Read the model definition and answer for the solid it produces. Units are mm, in the model's axes. Face numbers are marked on the shaded views. A direction names the side the tool comes from. Coordinates: 2 decimals unless noted, no trailing zeros. Loops run counter-clockwise (first coordinate to the right, second up) from the corner with the lowest first, then second, coordinate; pieces in that order, holes last.
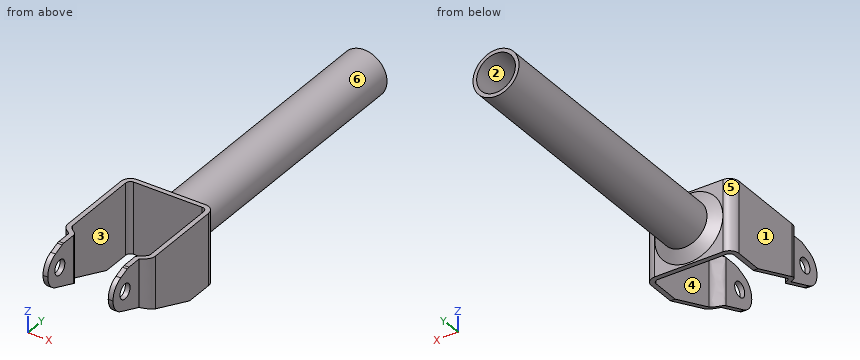
from build123d import *

# Parameters (mm, degrees)
EXTRUDE_THIN1_DEPTH = 38.1
CUT_EXTRUDE1_DEPTH  = 96.205221294
SKETCH5_R           = 3.96875
CUT_EXTRUDE2_DEPTH  = 96.205221294
SKETCH6_R           = 12.2936
SKETCH6_R_2         = 10.342534733
BOSS_EXTRUDE2_DEPTH = 152.4
SKETCH8_R           = 18.199007784
SKETCH7_R           = 10.342534733


# Read off the part's stored shape, not the designer's step: Extrude-Thin1
with BuildPart() as part:
    # Extrude-Thin1 outline → Extrude-Thin1 (new body)
    with BuildSketch(Plane.XY):
        with BuildLine():
            Line((-18.6817, 20.38347688), (-18.6817, 0))
            Line((-18.6817, 0), (-16.1417, 0))
            Line((-16.1417, 0), (-16.1417, 20.32))
            add(Edge.make_bspline(
                [(-20.8407, 26.67), (-20.8407, 23.763857752), (-15.646351535, 22.789211476), (-16.1417, 20.32)],
                knots=[0, 0, 0, 0, 1, 1, 1, 1], degree=3))
            Line((-20.8407, 26.67), (-20.8407, 68.58))
            ThreePointArc((-20.8407, 68.58), (-20.096751224, 70.376051224), (-18.3007, 71.12))
            Line((-18.3007, 71.12), (18.3007, 71.12))
            ThreePointArc((18.3007, 71.12), (20.096751224, 70.376051224), (20.8407, 68.58))
            Line((20.8407, 68.58), (20.8407, 26.67))
            add(Edge.make_bspline(
                [(16.1417, 20.32), (15.646351535, 22.789211476), (20.8407, 23.763857752), (20.8407, 26.67)],
                knots=[0, 0, 0, 0, 1, 1, 1, 1], degree=3))
            Line((16.1417, 20.32), (16.1417, 0))
            Line((16.1417, 0), (18.6817, 0))
            Line((18.6817, 0), (18.6817, 20.38347688))
            add(Edge.make_bspline(
                [(18.6817, 20.38347688), (18.765268898, 20.466690468), (18.888895007, 20.57668849), (19.198318415, 20.827254502), (19.383759179, 20.968114578), (19.796479851, 21.275209729), (20.023736725, 21.441568971), (20.503556211, 21.804901686), (20.7562224, 22.001844549), (21.272496014, 22.440788491), (21.53645688, 22.68275476), (22.056971887, 23.237206576), (22.314275473, 23.550298766), (22.782632726, 24.278317238), (22.993321794, 24.695356067), (23.294062312, 25.62890672), (23.3807, 26.144600529), (23.3807, 26.67)],
                knots=[0, 0, 0, 0, 0.125, 0.125, 0.25, 0.25, 0.375, 0.375, 0.5, 0.5, 0.625, 0.625, 0.75, 0.75, 0.875, 0.875, 1, 1, 1, 1], degree=3))
            Line((23.3807, 26.67), (23.3807, 68.58))
            ThreePointArc((23.3807, 68.58), (21.892802448, 72.172102448), (18.3007, 73.66))
            Line((18.3007, 73.66), (-18.3007, 73.66))
            ThreePointArc((-18.3007, 73.66), (-21.892802448, 72.172102448), (-23.3807, 68.58))
            Line((-23.3807, 68.58), (-23.3807, 26.67))
            add(Edge.make_bspline(
                [(-23.3807, 26.67), (-23.3807, 26.144600529), (-23.294062312, 25.62890672), (-22.993321794, 24.695356067), (-22.782632726, 24.278317238), (-22.314275473, 23.550298766), (-22.056971887, 23.237206576), (-21.53645688, 22.68275476), (-21.272496014, 22.440788491), (-20.7562224, 22.001844549), (-20.503556211, 21.804901686), (-20.023736725, 21.441568971), (-19.796479851, 21.275209729), (-19.383759179, 20.968114578), (-19.198318415, 20.827254502), (-18.888895007, 20.57668849), (-18.765268898, 20.466690468), (-18.6817, 20.38347688)],
                knots=[0, 0, 0, 0, 0.125, 0.125, 0.25, 0.25, 0.375, 0.375, 0.5, 0.5, 0.625, 0.625, 0.75, 0.75, 0.875, 0.875, 1, 1, 1, 1], degree=3))
        make_face()
    extrude(amount=EXTRUDE_THIN1_DEPTH)

    # Sketch3 → Cut-Extrude1 (cut, through all)
    with BuildSketch(Plane.ZY.offset(23.3807)):
        with BuildLine():
            Line((18.086653696, 6.133752432), (0, 53.604932722))
            Line((0, 53.604932722), (0, 0))
            Line((0, 0), (26.9875, 0))
            ThreePointArc((26.9875, 0), (21.582687704, 1.681937521), (18.086653696, 6.133752432))
        make_face()
        with BuildLine():
            ThreePointArc((35.888346304, 6.133752432), (32.392312296, 1.681937521), (26.9875, 0))
            Line((26.9875, 0), (38.1, 0))
            Line((38.1, 0), (38.1, 12.596443014))
            ThreePointArc((38.1, 12.596443014), (38.040956068, 11.949441708), (37.865774898, 11.323815275))
            Line((37.865774898, 11.323815275), (35.888346304, 6.133752432))
        make_face()
    extrude(amount=-CUT_EXTRUDE1_DEPTH, mode=Mode.SUBTRACT)

    # Sketch5 → Cut-Extrude2 (cut, through all)
    with BuildSketch(Plane.ZY.offset(23.3807)):
        with Locations((26.9875, 9.525)):
            Circle(SKETCH5_R)
    extrude(amount=-CUT_EXTRUDE2_DEPTH, mode=Mode.SUBTRACT)

    # Sketch6 → Boss-Extrude2 (add)
    with BuildSketch(Plane(origin=(0, 73.66, 0), x_dir=(1, 0, 0), z_dir=(0, 1, 0))):
        with Locations(Location((0, -19.05, 0), (0, 0, 90))):
            Circle(SKETCH6_R)
        with Locations(Location((0, -19.05, 0), (0, 0, 90))):
            Circle(SKETCH6_R_2, mode=Mode.SUBTRACT)
    extrude(amount=BOSS_EXTRUDE2_DEPTH)

    # Sketch8 → Loft2 section 0
    with BuildSketch(Plane(origin=(0, 73.66, 0), x_dir=(1, 0, 0), z_dir=(0, 1, 0))):
        with Locations((0, -19.05)):
            Circle(SKETCH8_R)
    # Sketch7 → Loft2 section 1
    with BuildSketch(Plane(origin=(0, 78.74, 0), x_dir=(1, 0, 0), z_dir=(0, 1, 0))):
        with Locations((0, -19.05)):
            Circle(SKETCH7_R)
    loft()


solid = part.part
Item 1: Determine the mould class of the marked faces 4, 5 and 6 for opening direction X: released by +X, released by -X, zero draft, split by the parting line, or undercut.
Numbers:
face 4: undercut
face 5: released by -X
face 6: split by the parting line
Item 2: A cutting plane is placed at B-B on y = 210. Determine the outline of the cut face in (x, z).
Numbers:
outline: circle Ø24.59 at (0, 19.05); hole circle Ø20.69 at (0, 19.05)
Item 3: Find the intervals of material crossed by line 1 along X through (y, z) = (138, 19.05); line 2 along X through (y, z) = (49.5, 2); line 3 along Z through (x, y) = (-2, 161.5), in increasing order.
Numbers:
line 1: x = -12.29 to -10.34, 10.34 to 12.29
line 2: x = -23.38 to -20.84, 20.84 to 23.38
line 3: z = 6.92 to 8.9, 29.2 to 31.18
Item 4: A cutting plane is placed at A-A on x = 0. Determine the outline of the cut face in (y, z).
Numbers:
outline: (71.12, 0) - (73.66, 0) - (73.66, 0.85) - (77.48, 6.76) - (226.06, 6.76) - (226.06, 8.71) - (78.74, 8.71) - (78.74, 29.39) - (226.06, 29.39) - (226.06, 31.34) - (77.48, 31.34) - (73.66, 37.25) - (73.66, 38.1) - (71.12, 38.1) - close
Item 5: Which of the six approach directions +Z, -Z, +X, -X, +Y, -Y give full straight-line access (tool end or side, diameter ignored) to the marked faces 1, 2 and 3?
Numbers:
face 1: +Z, -Z, -X, +Y, -Y
face 2: +Y
face 3: +Z, -Z
Item 6: Given pin 1 (10 mm diameter, centred on y = 11, z = 23.5, fed in from +X); pin 2 (10 mm diameter, centred on y = 5, z = 30.5, fed in from -X); pin 3 (3 mm diameter, centred on x = 9.5, z = 27.5, fed in from +Y); pin 4 (12 mm diameter, centred on y = 155, z = 30, fed in from +X), each flat-ended and moving along its own axis, determine where each tip first touches the part or whether it passes through.
Numbers:
pin 1: stops at x = 18.68
pin 2: stops at x = -18.68
pin 3: stops at y = 226.06
pin 4: stops at x = 11.25
